Geometry: final body of the model. Coordinates: model frame, mm. Face numbers are marked on the shaded views. A direction names the side the tool comes from. Give positions to 0.01 mm unless a question says otherwise; leave off trailing zeros. Order: outer loops, then holes, each group sorted by start corner. A loop starts at its lowest first (then second) coordinate and runs counter-clockwise, first axis right, second up. Notation, with made-up numbers: (4, 88) - (17, 88) arc R27 cw to (17, 120) - close; hole circle Ø3 at (-30.75, 63.5). An arc over 180 degrees is marked (long way). Put each result on its own line as item: value. Start each with the question number.
1. Mould query, pull axis X, two halves, no side actions, for the marked faces 5, 6 and 7. Classes: pulls with the +X half, pulls with the -X half, needs draft (parallel to the pull), parting line crosses it, or undercut.
2. Section B-B on z = 3. Return the cut outline in (x, y) (3 decimals), plus the area to 3 significant figures.
3. Section D-D on x = 47.5. Return the cut outline in (y, z), plus the area to 3 significant figures.
4. Ray query, line 1 along Z through (x, y) = (21, 1.25) (3 decimals); line 2 along X through (y, z) = (4.75, 0.5); line 3 along Z through (x, y) = (6, 2.75) (3 decimals). Return the intervals inside material, ascending. Write a range as from..to.
5. Section A-A on x = 8.5. Return the cut outline in (y, z) (3 decimals).
6. First-contact query: P1, Ø0.9, axis at y = 0.76, z = -13.56, coming from the -X side; P2, Ø5.5, axis at y = 3, z = -9.5, coming from the +X side; P3, Ø3.5, axis at y = 3, z = 7.5, coming from the +X side. Flat tips, straight axial feed; report the tip coordinate or a pass-through.
7. Section C-C on x = 29. Return the cut outline in (y, z) (3 decimals).
8. Set-up query: the marked faces 1, 2, 3 and 4. Return all of +Z, -Z, +X, -X, +Y, -Y with unobstructed straight access to the full face (end or side cutting, diameter ignored); none if empty.
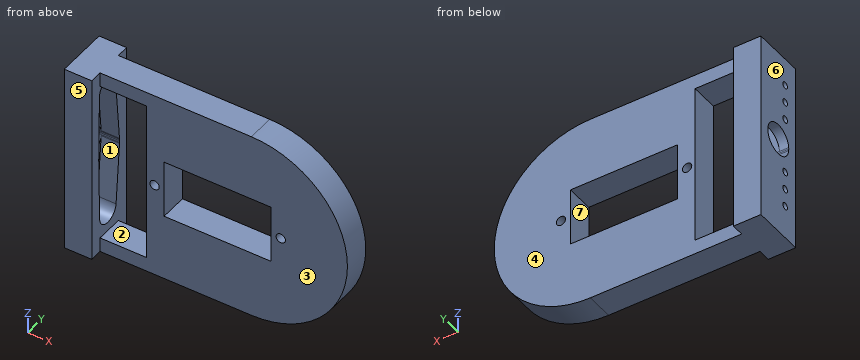
Autodesk Inventor part; units mm, degrees
ref_plane "YZ Plane" through (0, 0, 0) normal (1, 0, 0) x (0, 1, 0)
ref_plane "XZ Plane" through (0, 0, 0) normal (0, 1, 0) x (-1, 0, 0)
ref_plane "XY Plane" through (0, 0, 0) normal (0, 0, 1) x (1, 0, 0)
sketch "Sketch1" plane through (0, 0, 0) normal (0, 1, 0) x (-1, 0, 0)
  arc A0 (-33.02, 20.955) -> (-33.02, -20.955) centre (-33.02, 0) ccw
  line L0 (0, 20.955) -> (-33.02, 20.955)
  line L1 (-33.02, -20.955) -> (0, -20.955)
  line L2 (-13.979695, 6.35) -> (-37.347695, 6.35)
  line L3 (-37.347695, 6.35) -> (-37.347695, -6.35)
  line L4 (-37.347695, -6.35) -> (-13.979695, -6.35)
  line L5 (-13.979695, -6.35) -> (-13.979695, 6.35)
  circle A1 centre (-39.430495, 0) radius 1.016
  circle A2 centre (-11.896895, 0) radius 1.016
  line L6 (0, 20.955) -> (0, -20.955)
  point P0 (0, 0)
  point P1 (0, 0)
  point P2 (-37.347695, 0)
  dimension "d1" = 41.91
  dimension "d3" = 12.7
  dimension "d4" = 23.368
  dimension "d5" = 2.032
  dimension "d6" = 2.032
  dimension "d7" = 2.0828
  dimension "d8" = 2.0828
  dimension "d9" = 6.4105
  dimension "d87" = 33.02
  dimension "d88" = 33.02
extrude "Extrusion1" add sketch "Sketch1" along normal blind 6
sketch "Sketch4" plane through (0, 0, -20.955) normal (-1, 0, 0) x (0, 0, 1)
  line L0 (41.91, 8.715) -> (0, 8.715)
  line L1 (0, 8.715) -> (0, -2.715)
  line L2 (0, -2.715) -> (41.91, -2.715)
  line L3 (41.91, -2.715) -> (41.91, 8.715)
  line L4 (0, 0) -> (41.91, 0)
  line L5 (41.91, 0) -> (41.91, 6)
  point P0 (20.955, 0)
  point P1 (20.955, -2.715)
  point P2 (20.955, 0)
  point P3 (41.91, 3)
  point P4 (41.91, 3)
  dimension "d43" = 41.91
  dimension "d44" = 11.43
extrude "Extrusion4" add sketch "Sketch4" along normal blind 6
sketch "Sketch8" plane through (0, 6, 0) normal (0, 1, 0) x (1, 0, 0)
  line L0 (0, -17.78) -> (10.16, -17.78)
  line L1 (10.16, -17.78) -> (10.16, 17.78)
  line L2 (10.16, 17.78) -> (0, 17.78)
  line L3 (0, 17.78) -> (0, -17.78)
  line L4 (0, -20.955) -> (0, 20.955)
  point P0 (0, 0)
  point P1 (0, 0)
  point P2 (0, 0)
  point P3 (0, 0)
  point P4 (0, 0)
  point P5 (0, 0)
  dimension "d74" = 10.16
  dimension "d75" = 35.56
extrude "Extrusion10" cut sketch "Sketch8" against normal blind 16.999991
sketch "Sketch12" plane through (-6, 0, -20.955) normal (-1, 0, 0) x (0, 0, 1)
  line L0 (0, 8.715) -> (0, -2.715)
  line L1 (41.91, -2.715) -> (41.91, 8.715)
  arc A0 (35.512447, 0.300645) -> (35.512447, 5.699355) centre (35.37098, 3) ccw
  line L2 (21.59, -0.429) -> (35.512447, 0.300645)
  line L3 (21.59, 6.429) -> (35.512447, 5.699355)
  circle A1 centre (21.59, 3) radius 3.429
  line L4 (21.59, -0.429) -> (6.703499, 0.351168)
  line L5 (21.59, 6.429) -> (6.703499, 5.648832)
  arc A2 (6.703499, 5.648832) -> (6.703499, 0.351168) centre (6.842318, 3) ccw
  circle A3 centre (15.187051, 3) radius 0.75
  circle A4 centre (11.187051, 3) radius 0.75
  circle A5 centre (7.187051, 3) radius 0.75
  line L6 (21.59, 10.756719) -> (21.59, -4.756719)
  circle A6 centre (27.992949, 3) radius 0.75
  circle A7 centre (31.992949, 3) radius 0.75
  circle A8 centre (35.992949, 3) radius 0.75
  point P0 (34.925, 2)
  point P1 (34.925, 2)
  point P2 (34.925, 2)
  point P3 (14.859, -1.175)
  point P4 (14.859, 5.175)
  point P5 (34.925, 2)
  point P6 (41.91, 3)
  point P7 (38.07404, 3)
  point P8 (41.91, 3)
  point P9 (21.231572, 6.410216)
  point P10 (21.231572, -0.410216)
  point P11 (21.948428, -0.410216)
  point P12 (21.948428, 6.410216)
  point P13 (6.205131, 2.479358)
  point P14 (9.863981, 3)
  point P15 (5.48634, 2.396716)
  point P16 (4.189851, 3)
  point P17 (0, 3)
  point P18 (0, 3)
  point P19 (41.91, 3)
  dimension "d143" = 6
  dimension "d144" = 6.858
  dimension "d145" = 6
  dimension "d146" = 13.78098
  dimension "d147" = 20.32
  dimension "d156" = 1.5
  dimension "d157" = 1.5
  dimension "d158" = 1.5
  dimension "d159" = 4
  dimension "d160" = 4
  dimension "d161" = 2.9972
  dimension "d162" = 17.40015
sketch "Sketch12 outline for Extrusion13" plane through (-6, 0, -20.955) normal (-1, 0, 0) x (0, 0, 1)
  line L0 (21.59, 6.429) -> (21.231572, 6.410216)
  line L1 (21.948428, 6.410216) -> (21.59, 6.429)
  arc A0 (21.948428, -0.410216) -> (21.948428, 6.410216) centre (21.59, 3) ccw
  line L2 (21.59, -0.429) -> (21.948428, -0.410216)
  line L3 (21.231572, -0.410216) -> (21.59, -0.429)
  arc A1 (21.231572, 6.410216) -> (21.231572, -0.410216) centre (21.59, 3) ccw
extrude "Extrusion13" cut sketch "Sketch12 outline for Extrusion13" against normal blind 8.762492
sketch "Sketch17" plane through (0, 0, -20.955) normal (1, 0, 0) x (0, 0, -1)
  arc A0 (-7.753278, -0.143381) -> (-7.582189, 5.248432) centre (-7.80902, 2.557009) ccw
  line L0 (-21.59, -0.429) -> (-7.753278, -0.143381)
  line L1 (-21.59, 6.429) -> (-7.582189, 5.248432)
  circle A1 centre (-21.59, 3) radius 3.429
  line L2 (-21.59, -0.429) -> (-36.606269, -0.19851)
  line L3 (-21.59, 6.429) -> (-36.548101, 5.0886)
  arc A2 (-36.548101, 5.0886) -> (-36.606269, -0.19851) centre (-36.310948, 2.442116) ccw
  arc A3 (-21.231572, -0.410216) -> (-21.231572, 6.410216) centre (-21.59, 3) ccw
  circle A4 centre (-27.970676, 2.471347) radius 0.75
  circle A5 centre (-31.970676, 2.471347) radius 0.75
  circle A6 centre (-35.970676, 2.471347) radius 0.75
  line L4 (-21.59, 6.429) -> (-21.59, -0.429)
  circle A7 centre (-15.209324, 2.471347) radius 0.75
  circle A8 centre (-11.209324, 2.471347) radius 0.75
  circle A9 centre (-7.209324, 2.471347) radius 0.75
  point P0 (-20.955, 0)
  point P1 (-16.352581, -1.161112)
  point P2 (-16.352581, 5.188888)
  point P3 (-5.109414, 2.471347)
  point P4 (-21.695241, -0.427385)
  point P5 (-22.199652, 6.374369)
  point P6 (-21.016089, 6.380631)
  point P7 (-21.448497, -0.426079)
  point P8 (-30.453399, 2.232188)
  point P9 (-26.794548, 2.471347)
  point P10 (-31.172189, 2.149546)
  point P11 (-38.967876, 2.471347)
  dimension "d150" = 6
  dimension "d151" = 6.858
  dimension "d152" = 6
  dimension "d153" = 13.78098
  dimension "d163" = 1.5
  dimension "d164" = 1.5
  dimension "d165" = 1.5
  dimension "d166" = 4
  dimension "d167" = 4
  dimension "d168" = 2.9972
sketch "Sketch17 outline for Extrusion17" plane through (0, 0, -20.955) normal (1, 0, 0) x (0, 0, -1)
  arc A0 (-36.548101, 5.0886) -> (-36.606269, -0.19851) centre (-36.310948, 2.442116) ccw
  line L0 (-22.199652, 6.374369) -> (-36.548101, 5.0886)
  arc A1 (-21.695241, -0.427385) -> (-22.199652, 6.374369) centre (-21.59, 3) cw
  line L1 (-36.606269, -0.19851) -> (-21.695241, -0.427385)
  arc A2 (-7.753278, -0.143381) -> (-7.582189, 5.248432) centre (-7.80902, 2.557009) ccw
  line L2 (-21.448497, -0.426079) -> (-7.753278, -0.143381)
  arc A3 (-21.016089, 6.380631) -> (-21.448497, -0.426079) centre (-21.59, 3) cw
  line L3 (-7.582189, 5.248432) -> (-21.016089, 6.380631)
extrude "Extrusion17" cut sketch "Sketch17 outline for Extrusion17" against normal blind 4
sketch "Sketch19" plane through (-4, 0, -20.955) normal (1, 0, 0) x (0, 0, -1)
  circle A0 centre (-27.7378, 0.757495) radius 0.75
  circle A1 centre (-31.7378, 0.757495) radius 0.75
  circle A2 centre (-35.7378, 0.757495) radius 0.75
  line L0 (-38.735, 6) -> (-38.735, 3.530276)
  line L1 (-21.564652, 3.265138) -> (-21.564652, -1.203525)
  circle A3 centre (-15.391504, 0.757495) radius 0.75
  circle A4 centre (-11.391504, 0.757495) radius 0.75
  circle A5 centre (-7.391504, 0.757495) radius 0.75
  point P0 (-20.955, 0)
  point P1 (-32.395372, 0.835812)
  point P2 (-31.71002, 0.757495)
  point P3 (-38.735, 1.75317)
  point P4 (-38.735, 4.765138)
  dimension "d169" = 1.5
  dimension "d170" = 1.5
  dimension "d171" = 1.5
  dimension "d172" = 4
  dimension "d173" = 4
  dimension "d174" = 2.9972
extrude "Extrusion18" cut sketch "Sketch19" against normal blind 25.4
properties part number "unions2s3pt"
Resolved:
1. face 5: needs draft
1. face 6: pulls with the -X half
1. face 7: undercut
2. outline: (-6, -2.715) - (0, -2.715) - (0, -0.393) - (-4, -0.393) - (-4, 0.517) - (-6, 0.517) - close; (-6, 5.483) - (-4, 5.483) - (-4, 6.217) - (0, 6.217) - (0, 8.715) - (-6, 8.715) - close; (10.16, 0) - (13.98, 0) - (13.98, 6) - (10.16, 6) - close; (37.348, 0) - (53.759, 0) - (53.759, 6) - (37.348, 6) - close
2. area: 154 mm^2
3. outline: (0, -15.15) - (6, -15.15) - (6, 15.15) - (0, 15.15) - close
3. area: 182 mm^2
4. line 1: -20.955..-6.35, 6.35..20.955
4. line 2: 10.16..11.01, 12.78..13.98, 37.35..38.55, 40.31..53.97
4. line 3: -20.955..-17.78, 17.78..20.955
5. outline: (0, -20.955) - (6, -20.955) - (6, -17.78) - (0, -17.78) - close; (0, 17.78) - (6, 17.78) - (6, 20.955) - (0, 20.955) - close
6. P1: x = 10.16
6. P2: x = 52.86
6. P3: x = 53.17
7. outline: (0, -20.955) - (6, -20.955) - (6, -6.35) - (0, -6.35) - close; (0, 6.35) - (6, 6.35) - (6, 20.955) - (0, 20.955) - close
8. face 1: none
8. face 2: +Y, -Y
8. face 3: +Z, -Z, +X, -Y
8. face 4: +Z, -Z, +X, +Y
